```python
from build123d import *

# Parameters (mm, degrees)
EXTRUDE_1_DEPTH     = 1.5
CUT_EXTRUDE_1_REACH = 5
SKETCH_2_R          = 1.6
SKETCH_3_R          = 2
CUT_EXTRUDE_2_DEPTH = 10


with BuildPart() as part:
    # 草图1 → 凸台-拉伸1 (new body, symmetric)
    with BuildSketch(Plane.XY):
        with BuildLine():
            Line((32.2, 68.7), (34.8, 68.7))
            ThreePointArc((34.8, 68.7), (34.941421356, 68.758578644), (35, 68.9))
            Line((35, 68.9), (35, 70.15))
            ThreePointArc((35, 70.15), (35.146446609, 70.503553391), (35.5, 70.65))
            Line((35.5, 70.65), (37.5, 70.65))
            ThreePointArc((37.5, 70.65), (37.853553391, 70.503553391), (38, 70.15))
            Line((38, 70.15), (38, 44.35))
            ThreePointArc((38, 44.35), (37.853553391, 43.996446609), (37.5, 43.85))
            Line((37.5, 43.85), (35.5, 43.85))
            ThreePointArc((35.5, 43.85), (35.146446609, 43.996446609), (35, 44.35))
            Line((35, 44.35), (35, 45.6))
            ThreePointArc((35, 45.6), (34.941421356, 45.741421356), (34.8, 45.8))
            Line((34.8, 45.8), (32.2, 45.8))
            ThreePointArc((32.2, 45.8), (32.058578644, 45.741421356), (32, 45.6))
            Line((32, 45.6), (32, -45.6))
            ThreePointArc((32, -45.6), (32.058578644, -45.741421356), (32.2, -45.8))
            Line((32.2, -45.8), (34.8, -45.8))
            ThreePointArc((34.8, -45.8), (34.941421356, -45.741421356), (35, -45.6))
            Line((35, -45.6), (35, -44.35))
            ThreePointArc((35, -44.35), (35.146446609, -43.996446609), (35.5, -43.85))
            Line((35.5, -43.85), (37.5, -43.85))
            ThreePointArc((37.5, -43.85), (37.853553391, -43.996446609), (38, -44.35))
            Line((38, -44.35), (38, -70.15))
            ThreePointArc((38, -70.15), (37.853553391, -70.503553391), (37.5, -70.65))
            Line((37.5, -70.65), (35.5, -70.65))
            ThreePointArc((35.5, -70.65), (35.146446609, -70.503553391), (35, -70.15))
            Line((35, -70.15), (35, -68.9))
            ThreePointArc((35, -68.9), (34.941421356, -68.758578644), (34.8, -68.7))
            Line((34.8, -68.7), (32.2, -68.7))
            ThreePointArc((32.2, -68.7), (32.058578644, -68.758578644), (32, -68.9))
            Line((32, -68.9), (32, -72))
            ThreePointArc((32, -72), (31.121320344, -74.121320344), (29, -75))
            Line((29, -75), (-29, -75))
            ThreePointArc((-29, -75), (-31.121320344, -74.121320344), (-32, -72))
            Line((-32, -72), (-32, -68.9))
            ThreePointArc((-32, -68.9), (-32.058578644, -68.758578644), (-32.2, -68.7))
            Line((-32.2, -68.7), (-34.8, -68.7))
            ThreePointArc((-34.8, -68.7), (-34.941421356, -68.758578644), (-35, -68.9))
            Line((-35, -68.9), (-35, -70.15))
            ThreePointArc((-35, -70.15), (-35.146446609, -70.503553391), (-35.5, -70.65))
            Line((-35.5, -70.65), (-37.5, -70.65))
            ThreePointArc((-37.5, -70.65), (-37.853553391, -70.503553391), (-38, -70.15))
            Line((-38, -70.15), (-38, -44.35))
            ThreePointArc((-38, -44.35), (-37.853553391, -43.996446609), (-37.5, -43.85))
            Line((-37.5, -43.85), (-35.5, -43.85))
            ThreePointArc((-35.5, -43.85), (-35.146446609, -43.996446609), (-35, -44.35))
            Line((-35, -44.35), (-35, -45.6))
            ThreePointArc((-35, -45.6), (-34.941421356, -45.741421356), (-34.8, -45.8))
            Line((-34.8, -45.8), (-32.2, -45.8))
            ThreePointArc((-32.2, -45.8), (-32.058578644, -45.741421356), (-32, -45.6))
            Line((-32, -45.6), (-32, 45.6))
            ThreePointArc((-32, 45.6), (-32.058578644, 45.741421356), (-32.2, 45.8))
            Line((-32.2, 45.8), (-34.8, 45.8))
            ThreePointArc((-34.8, 45.8), (-34.941421356, 45.741421356), (-35, 45.6))
            Line((-35, 45.6), (-35, 44.35))
            ThreePointArc((-35, 44.35), (-35.146446609, 43.996446609), (-35.5, 43.85))
            Line((-35.5, 43.85), (-37.5, 43.85))
            ThreePointArc((-37.5, 43.85), (-37.853553391, 43.996446609), (-38, 44.35))
            Line((-38, 44.35), (-38, 70.15))
            ThreePointArc((-38, 70.15), (-37.853553391, 70.503553391), (-37.5, 70.65))
            Line((-37.5, 70.65), (-35.5, 70.65))
            ThreePointArc((-35.5, 70.65), (-35.146446609, 70.503553391), (-35, 70.15))
            Line((-35, 70.15), (-35, 68.9))
            ThreePointArc((-35, 68.9), (-34.941421356, 68.758578644), (-34.8, 68.7))
            Line((-34.8, 68.7), (-32.2, 68.7))
            ThreePointArc((-32.2, 68.7), (-32.058578644, 68.758578644), (-32, 68.9))
            Line((-32, 68.9), (-32, 72))
            ThreePointArc((-32, 72), (-31.121320344, 74.121320344), (-29, 75))
            Line((-29, 75), (29, 75))
            ThreePointArc((29, 75), (31.121320344, 74.121320344), (32, 72))
            Line((32, 72), (32, 68.9))
            ThreePointArc((32, 68.9), (32.058578644, 68.758578644), (32.2, 68.7))
        make_face()
    extrude(amount=EXTRUDE_1_DEPTH, both=True)

    # 草图2 → 切除-拉伸1 (cut, up to next)
    with BuildSketch(Plane(origin=(0, 0, -1.5), x_dir=(-1, 0, 0), z_dir=(0, 0, -1)), mode=Mode.PRIVATE) as cut_extrude_1_sk1:
        with Locations((23.8, 8.34)):
            Circle(SKETCH_2_R)
    cut_extrude_1_tool1 = extrude(cut_extrude_1_sk1.sketch, amount=-CUT_EXTRUDE_1_REACH, mode=Mode.PRIVATE) & part.part
    add(cut_extrude_1_tool1.solids().sort_by_distance((-23.8, 8.34, -1.5))[0], mode=Mode.SUBTRACT)
    # 草图2 → 切除-拉伸1 (cut, up to next)
    with BuildSketch(Plane(origin=(0, 0, -1.5), x_dir=(-1, 0, 0), z_dir=(0, 0, -1)), mode=Mode.PRIVATE) as cut_extrude_1_sk2:
        with Locations((8.56, -42.46)):
            Circle(SKETCH_2_R)
    cut_extrude_1_tool2 = extrude(cut_extrude_1_sk2.sketch, amount=-CUT_EXTRUDE_1_REACH, mode=Mode.PRIVATE) & part.part
    add(cut_extrude_1_tool2.solids().sort_by_distance((-8.56, -42.46, -1.5))[0], mode=Mode.SUBTRACT)
    # 草图2 → 切除-拉伸1 (cut, up to next)
    with BuildSketch(Plane(origin=(0, 0, -1.5), x_dir=(-1, 0, 0), z_dir=(0, 0, -1)), mode=Mode.PRIVATE) as cut_extrude_1_sk3:
        with Locations((-19.38, -42.46)):
            Circle(SKETCH_2_R)
    cut_extrude_1_tool3 = extrude(cut_extrude_1_sk3.sketch, amount=-CUT_EXTRUDE_1_REACH, mode=Mode.PRIVATE) & part.part
    add(cut_extrude_1_tool3.solids().sort_by_distance((19.38, -42.46, -1.5))[0], mode=Mode.SUBTRACT)
    # 草图2 → 切除-拉伸1 (cut, up to next)
    with BuildSketch(Plane(origin=(0, 0, -1.5), x_dir=(-1, 0, 0), z_dir=(0, 0, -1)), mode=Mode.PRIVATE) as cut_extrude_1_sk4:
        with Locations((-24.46, 9.61)):
            Circle(SKETCH_2_R)
    cut_extrude_1_tool4 = extrude(cut_extrude_1_sk4.sketch, amount=-CUT_EXTRUDE_1_REACH, mode=Mode.PRIVATE) & part.part
    add(cut_extrude_1_tool4.solids().sort_by_distance((24.46, 9.61, -1.5))[0], mode=Mode.SUBTRACT)

    # 草图3 → 切除-拉伸2 (cut)
    with BuildSketch(Plane.XY.offset(1.5)):
        with Locations((14, 26)):
            Circle(SKETCH_3_R)
        with Locations((14, -26)):
            Circle(SKETCH_3_R)
        with Locations((-14, 26)):
            Circle(SKETCH_3_R)
        with Locations((-14, -26)):
            Circle(SKETCH_3_R)
    extrude(amount=-CUT_EXTRUDE_2_DEPTH, mode=Mode.SUBTRACT)


solid = part.part
```
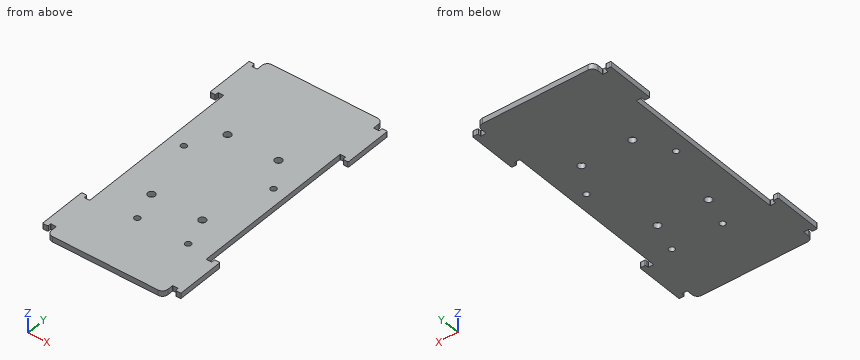
Model file for the job. Use its own axes, mm. Coordinates: 2 decimals unless noted, no trailing zeros. Order: outer loops, then holes, each group sorted by start corner. A loop starts at its lowest first (then second) coordinate and runs counter-clockwise, first axis right, second up. Notation, with made-up numbers: (56, 36.25) - (98, 36.25) arc R20 ccw to (98, 68.25) - close; hole circle Ø11 at (28, 55.25). An arc over 180 degrees is marked (long way). Return JSON: item names as keys, results as strings. Group by question number.
1) Probe line 1 (Y direction, x = -14, z = 0.9); line 2 (Y direction, x = -33, z = 1.1); line 3 (Y direction, x = -8.56, z = 0.05). List the from-to ranges inside material, lowest first. Write a range as from..to.
2) Saw through at B-B, the plane y = 26. Write the cut outline in (x, z), plus the area to 3 significant figures.
3) Flat gauge pins, fed straight in: P1, Ø0.6, axis at x = -37, z = 0.5, coming from the -Y side; P2, Ø1.3, axis at x = 33.5, z = -0.5, coming from the +Y side; P3, Ø1.6, axis at x = -37, z = 0.5, coming from the +Y side. Where does each tip first touch, or does it go through?
4) Saw through at C-C, the plane z = -0.6. Count the separate pieces of the cut face and the enclosed holes in it, plus the area to 3 significant figures.
5) Saw through at D-D, the plane y = -16. Write the cut outline in (x, z).
6) Saw through at A-A, the plane x = -14. Write the cut outline in (y, z), plus the area to 3 significant figures.
Values found:
{
 "1": {"line 1": "y = -75..-28, -24..24, 28..75", "line 2": "y = -68.7..-45.8, 45.8..68.7", "line 3": "y = -75..-44.06, -40.86..75"},
 "2": {"outline": "(-32, -1.5) - (-16, -1.5) - (-16, 1.5) - (-32, 1.5) - close; (-12, -1.5) - (12, -1.5) - (12, 1.5) - (-12, 1.5) - close; (16, -1.5) - (32, -1.5) - (32, 1.5) - (16, 1.5) - close", "area": "168 mm²"},
 "3": {"P1": "stops at y = -70.65", "P2": "stops at y = 68.7", "P3": "stops at y = 70.65"},
 "4": {"separate pieces": "1", "enclosed holes": "8", "area": "10,100 mm²"},
 "5": {"outline": "(-32, -1.5) - (32, -1.5) - (32, 1.5) - (-32, 1.5) - close"},
 "6": {"outline": "(-75, -1.5) - (-28, -1.5) - (-28, 1.5) - (-75, 1.5) - close; (-24, -1.5) - (24, -1.5) - (24, 1.5) - (-24, 1.5) - close; (28, -1.5) - (75, -1.5) - (75, 1.5) - (28, 1.5) - close", "area": "426 mm²"}
}
